For this review, take the finished solid that the model builds, in its own axes (mm). A direction names the side the tool comes from. Round coordinates to 2 decimals unless told otherwise and drop trailing zeros. Loops run counter-clockwise (first coordinate to the right, second up) from the corner with the lowest first, then second, coordinate; pieces in that order, holes last.
1) Insertion check: pin 1 (1.2 mm diameter, centred on y = 26.5, z = 2.5, fed in from -X); pin 2 (0.8 mm diameter, centred on x = 51, z = 2.5, fed in from -Y); pin 3 (1.6 mm diameter, centred on x = 51, z = 2, fed in from +Y). Each pin has a flat end and moves straight along its axis. Give the tip position at first contact, or say it passes through.
2) Wall thickness on L1, parallel to Y at x = 47.5, z = 0.85; L2, parallel to X at y = 20.5, z = 1.7; L3, parallel to Y at x = 6.5, z = 0.6: over which ranges is each line inside the solid? List them lowest first.
3) Take a section at A-A (z = 2.4). State the section outline as (x, y) points.
4) Take a section at C-C (x = 35.5). State the section outline as (y, z) points, then the cut area to 3 significant figures.
5) Take a section at B-B (y = 16.5). State the section outline as (x, z) points.
6) Tool access review of faces 1 (the flat face through (24, 40.25, 3)), 2 (the flat face through (50, 43.25, 2)), 3 (the flat face through (50, 24, 3.1)), 4 (the flat face through (1.3, 23, 3)): name each direction out of +Z, -Z, +X, -X, +Y, -Y from which nothing blocks a thin tool from reaching the whole face with its end or side.
7) Take a section at D-D (x = 6.5). State the section outline as (y, z) points.
```python
from build123d import *

# Parameters (mm, degrees)
ESQUISSE1_W             = 51.5
ESQUISSE1_H             = 46.5
BOSS_EXTRU_1_DEPTH      = 1.6
ESQUISSE2_W             = 46
ESQUISSE2_H             = 34
BOSS_EXTRU_2_DEPTH      = 2.5
ESQUISSE3_W             = 2.5
ESQUISSE3_H             = 40
BOSS_EXTRU_3_DEPTH      = 1.5
ESQUISSE4_R             = 1.5
ENL_V_MAT_EXTRU_1_DEPTH = 70.431621038
CONG_1_R                = 3


with BuildPart() as part:
    # Esquisse1 → Boss.-Extru.1 (new body)
    with BuildSketch(Plane.XY):
        with Locations((25.75, 23.25)):
            Rectangle(ESQUISSE1_W, ESQUISSE1_H)
    extrude(amount=BOSS_EXTRU_1_DEPTH)

    # Esquisse2 → Boss.-Extru.2 (add)
    with BuildSketch(Plane.XY.offset(1.6)):
        with Locations((24.3, 23.25)):
            Rectangle(ESQUISSE2_W, ESQUISSE2_H)
    extrude(amount=BOSS_EXTRU_2_DEPTH)

    # Esquisse3 → Boss.-Extru.3 (add)
    with BuildSketch(Plane.XY.offset(1.6)):
        with Locations((50.25, 23.25)):
            Rectangle(ESQUISSE3_W, ESQUISSE3_H)
    extrude(amount=BOSS_EXTRU_3_DEPTH)

    # Esquisse4 → Enlèv. mat.-Extru.1 (cut, through all)
    with BuildSketch(Plane.XY.offset(1.6)):
        with Locations((47.5, 3.25)):
            Circle(ESQUISSE4_R)
        with Locations((47.5, 43.25)):
            Circle(ESQUISSE4_R)
        with Locations((6.5, 3.25)):
            Circle(ESQUISSE4_R)
    extrude(amount=-ENL_V_MAT_EXTRU_1_DEPTH, mode=Mode.SUBTRACT)

    # Congé1
    cong_1_edges = [part.edges().sort_by_distance(p)[0] for p in [
        (0, 46.5, 0.8),
        (51.5, 46.5, 0.8),
        (51.5, 0, 0.8),
        (0, 0, 0.8),
    ]]
    fillet(cong_1_edges, radius=CONG_1_R)


solid = part.part
```
Response:
1. pin 1: stops at x = 1.3
1. pin 2: stops at y = 3.25
1. pin 3: stops at y = 45.89
2. L1: y = 0 to 1.75, 4.75 to 41.75, 44.75 to 46.5
2. L2: x = 1.3 to 47.3, 49 to 51.5
2. L3: y = 0 to 1.75, 4.75 to 46.5
3. outline: (1.3, 6.25) - (47.3, 6.25) - (47.3, 40.25) - (1.3, 40.25) - close; (49, 3.25) - (51.5, 3.25) - (51.5, 43.25) - (49, 43.25) - close
4. outline: (0, 0) - (46.5, 0) - (46.5, 1.6) - (40.25, 1.6) - (40.25, 4.1) - (6.25, 4.1) - (6.25, 1.6) - (0, 1.6) - close
4. area: 159 mm2
5. outline: (0, 0) - (51.5, 0) - (51.5, 3.1) - (49, 3.1) - (49, 1.6) - (47.3, 1.6) - (47.3, 4.1) - (1.3, 4.1) - (1.3, 1.6) - (0, 1.6) - close
6. face 1: +Z, -X, +Y
6. face 2: +Z, +X, -X, +Y
6. face 3: +Z, +X, +Y, -Y
6. face 4: +Z, -X, +Y, -Y
7. outline: (0, 0) - (1.75, 0) - (1.75, 1.6) - (0, 1.6) - close; (4.75, 0) - (46.5, 0) - (46.5, 1.6) - (40.25, 1.6) - (40.25, 4.1) - (6.25, 4.1) - (6.25, 1.6) - (4.75, 1.6) - close
